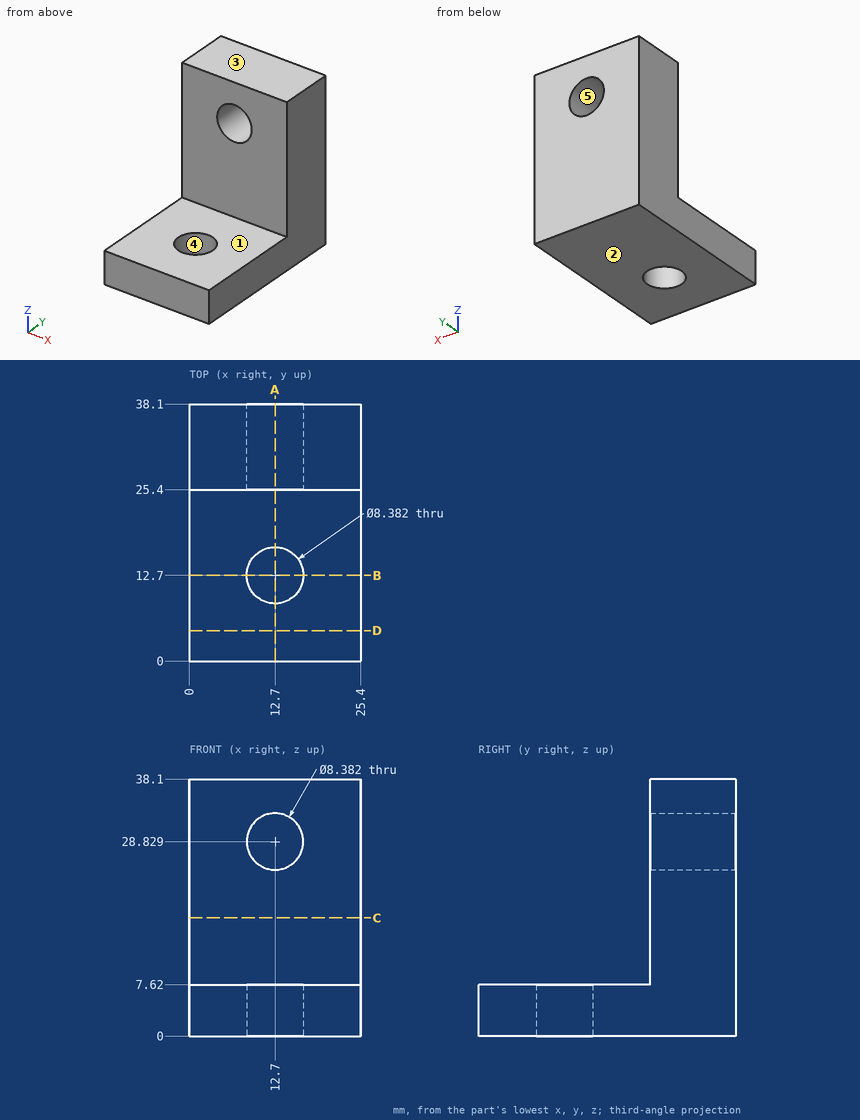
Answer from the drawing. Dimensions are ordinates in mm from the lowest x, y and z of the part. A direction names the side the tool comes from. Coordinates: 2 decimals unless noted, no trailing zeros. Loops run counter-clockwise (first coordinate to the right, second up) from the corner with the lowest first, then second, coordinate; pieces in that order, holes last.
1) Section D-D (y = 4.5) is taken. Give the vertices of the cut face in (x, z), plus the area to 3 significant figures.
Results:
outline: (0, 0) - (25.4, 0) - (25.4, 7.62) - (0, 7.62) - close
area: 194 mm2
2) For the marked faces 1 and 2, determine the directions among +Z, -Z, +X, -X, +Y, -Y from which every point of the face is accessible in a straight line to the end or side of a thin tool.
Results:
face 1: +Z, +X, -X, -Y
face 2: -Z, +X, -X, +Y, -Y
3) A flat-ended cylindrical pin translates along its axis: pin 1 (7.5 mm diameter, centred on x = 12, z = 18, fed in from -Y). Find the tip coordinate at first contact, or state that the pin passes through.
Results:
pin 1: stops at y = 25.4
4) Section C-C (z = 17.5) is taken. Give the vertices of the cut face in (x, y), plus the area to 3 significant figures.
Results:
outline: (0, 25.4) - (25.4, 25.4) - (25.4, 38.1) - (0, 38.1) - close
area: 323 mm2
5) Section A-A (x = 12.7) is taken. Give the vertices of the cut face in (y, z), plus the area to 3 significant figures.
Results:
outline: (0, 0) - (8.51, 0) - (8.51, 7.62) - (0, 7.62) - close; (16.89, 0) - (38.1, 0) - (38.1, 24.64) - (25.4, 24.64) - (25.4, 7.62) - (16.89, 7.62) - close; (25.4, 33.02) - (38.1, 33.02) - (38.1, 38.1) - (25.4, 38.1) - close
area: 507 mm2
6) Section B-B (y = 12.7) is taken. Give the vertices of the cut face in (x, z), plus the area to 3 significant figures.
Results:
outline: (0, 0) - (8.51, 0) - (8.51, 7.62) - (0, 7.62) - close; (16.89, 0) - (25.4, 0) - (25.4, 7.62) - (16.89, 7.62) - close
area: 130 mm2
7) For a pull along Z with two mould halves and no side action, classify the marked faces 3, 4 and 5 as +Z half, -Z half, draft (parallel to the pull), parting line (faces both ways), or undercut.
Results:
face 3: +Z half
face 4: draft
face 5: undercut
8) Consider probe 1 along Y at (x, z) = (12.7, 5.75); probe 2 along Z at (x, y) = (12.7, 32.25); probe 3 along Z at (x, y) = (18, 22). Determine where each line is inside the solid, lowest interval first.
Results:
probe 1: y = 0 to 8.51, 16.89 to 38.1
probe 2: z = 0 to 24.64, 33.02 to 38.1
probe 3: z = 0 to 7.62
